Build history of the part. All positions in model axes, mm. A direction names the side the tool comes from. Round coordinates to 2 decimals unless told otherwise and drop trailing zeros. Loops run counter-clockwise (first coordinate to the right, second up) from the corner with the lowest first, then second, coordinate; pieces in that order, holes last.
from build123d import *

# Parameters (mm, degrees)
SKETCH1_W           = 55
SKETCH1_H           = 30
SKETCH1_R           = 10.5
SKETCH1_W_2         = 12
SKETCH1_H_2         = 21
BOSS_EXTRUDE1_DEPTH = 7
SKETCH1_3_W         = 58.132008701
SKETCH1_3_H         = 32.587347793
SKETCH1_3_W_2       = 55
SKETCH1_3_H_2       = 30
BOSS_EXTRUDE2_DEPTH = 1


with BuildPart() as part:
    # Sketch1 → Boss-Extrude1 (new body)
    with BuildSketch(Plane(origin=(0, 0, 0), x_dir=(1, 0, 0), z_dir=(0, 1, 0))):
        Rectangle(SKETCH1_W, SKETCH1_H)
        with Locations(Location((13.99341574, 0, 0), (0, 0, 270))):
            Circle(SKETCH1_R, mode=Mode.SUBTRACT)
        with Locations((-14.212711625, -0.088861689)):
            Rectangle(SKETCH1_W_2, SKETCH1_H_2, mode=Mode.SUBTRACT)
    extrude(amount=-BOSS_EXTRUDE1_DEPTH)

    # Sketch1_3 → Boss-Extrude2 (add)
    with BuildSketch(Plane(origin=(0, 0, 0), x_dir=(1, 0, 0), z_dir=(0, 1, 0))):
        with Locations((0.128352579, -0.130903876)):
            Rectangle(SKETCH1_3_W, SKETCH1_3_H)
        Rectangle(SKETCH1_3_W_2, SKETCH1_3_H_2, mode=Mode.SUBTRACT)
    extrude(amount=-BOSS_EXTRUDE2_DEPTH)


solid = part.part
(1) Pin check, flat tips, straight feed: P1, Ø1.5, axis at x = 12, y = -4.5, coming from the -Z side; P2, Ø12, axis at x = 12.5, z = -12.5, coming from the +Y side; P3, Ø1.5, axis at y = -2, z = -10.5, coming from the -X side; P4, Ø1.8, axis at y = -4.5, z = 7, coming from the +X side. Stop position of each tip, or through.
Responses:
P1: stops at z = -15
P2: stops at y = 0
P3: stops at x = -27.5
P4: stops at x = 27.5
(2) Slice it at C-C on y = -3. List the corners of the cut face in (x, z).
Responses:
outline: (-27.5, -15) - (27.5, -15) - (27.5, 15) - (-27.5, 15) - close; hole (-20.21, -10.41) - (-8.21, -10.41) - (-8.21, 10.59) - (-20.21, 10.59) - close; hole circle Ø21 at (13.99, 0)
(3) Which spindle directions (+Z, -Z, +X, -X, +Y, -Y) get a long thin tool onto all of the face, cutting with end or side? Do faces 1 (the face through (-27.5, -4, 0)), 2 (the face through (0, 0, 0)), 3 (the face through (-14, -3, -10.411)), 4 (the face through (0, -7, 0)), 5 (the face through (27.5, -4, 0)). Say none if no direction does.
Responses:
face 1: +Z, -Z, -X, -Y
face 2: +Z, -Z, +X, -X, +Y
face 3: +Y, -Y
face 4: +Z, -Z, +X, -X, -Y
face 5: +Z, -Z, +X, -Y
(4) Slice it at D-D on x = -25. List the corners of the cut face in (y, z), plus the area to 3 significant figures.
Responses:
outline: (-7, -15) - (-1, -15) - (-1, -16.16) - (0, -16.16) - (0, 16.42) - (-1, 16.42) - (-1, 15) - (-7, 15) - close
area: 213 mm2
(5) Pull direction Z, two halves, no side cores. Call faces 6 (the face through (0, -4, 15)), 7 (the face through (-2, -1, 16)), 8 (the face through (-20.213, -3, 0)), 9 (the face through (0, -4, -15)): +Z half, -Z half, draft (parallel to the pull), parting line (faces both ways), or undercut.
Responses:
face 6: +Z half
face 7: draft
face 8: undercut
face 9: -Z half
(6) Slice it at B-B on x = -17.5. List the corners of the cut face in (y, z), plus the area to 3 significant figures.
Responses:
outline: (-7, -15) - (-1, -15) - (-1, -16.16) - (0, -16.16) - (0, -10.41) - (-7, -10.41) - close; (-7, 10.59) - (0, 10.59) - (0, 16.42) - (-1, 16.42) - (-1, 15) - (-7, 15) - close
area: 65.6 mm2
(7) Probe line 1 (X direction, y = -4.25, z = 0); line 2 (X direction, y = -4.25, z = 6.5); line 3 (Z direction, x = -19, y = -6). List the from-to ranges inside material, lowest first.
Responses:
line 1: x = -27.5 to -20.21, -8.21 to 3.49, 24.49 to 27.5
line 2: x = -27.5 to -20.21, -8.21 to 5.75, 22.24 to 27.5
line 3: z = -15 to -10.41, 10.59 to 15
(8) Slice it at A-A on z = 0. List the corners of the cut face in (x, y), plus the area to 3 significant figures.
Responses:
outline: (-28.94, -1) - (-27.5, -1) - (-27.5, -7) - (-20.21, -7) - (-20.21, 0) - (-28.94, 0) - close; (-8.21, -7) - (3.49, -7) - (3.49, 0) - (-8.21, 0) - close; (24.49, -7) - (27.5, -7) - (27.5, -1) - (29.19, -1) - (29.19, 0) - (24.49, 0) - close
area: 157 mm2
